Answer from the drawing. Dimensions are ordinates in mm from the lowest x, y and z of the part. Coordinates: 2 decimals unless noted, no trailing zeros. Write each loop counter-clockwise with the first axis right and the second up, starting at its lowest first coordinate (ties: lowest second). Pieces come first, ordered by that corner, then holes. Notation, with made-up numbers: (80, 1.25) - (91, 1.25) arc R32 ccw to (91, 30.25) - close; hole circle Ø1 at (83, -36.5). An arc over 180 degrees is marked (long way). Use one line per item in the form item = value. Start each with the question number.
Item 1: A cutting plane is placed at A-A (x = 38.1). Write down the section's boundary in (y, z).
Item 2: Given pin 1 (4 mm diameter, centred on x = 14, y = 26, fed in from -Z); pin 2 (3 mm diameter, centred on x = 67, z = 11, fed in from -Y); pin 3 (6 mm diameter, centred on x = 45, z = 32, fed in from +Y); pin 4 (12 mm diameter, centred on y = 47.5, z = 14, fed in from -X), each flat-ended and moving along its own axis, determine where each tip first touches the part or whether it passes through.
Item 3: A cutting plane is placed at B-B (z = 6). Write down the section's boundary in (x, y).
Item 4: Determine the mould class of the marked faces 1, 2 and 3 for opening direction X: released by +X, released by -X, zero draft, split by the parting line, or undercut.
Item 5: Consider probe 1 along Z at (x, y) = (23.5, 39); probe 2 along X at (y, z) = (38, 59); probe 3 along Y at (x, z) = (38.1, 60.25). Determine where each line is inside the solid, lowest interval first.
Item 6: A cutting plane is placed at C-C (z = 35). Write down the section's boundary in (x, y), then the cut area to 3 significant figures.
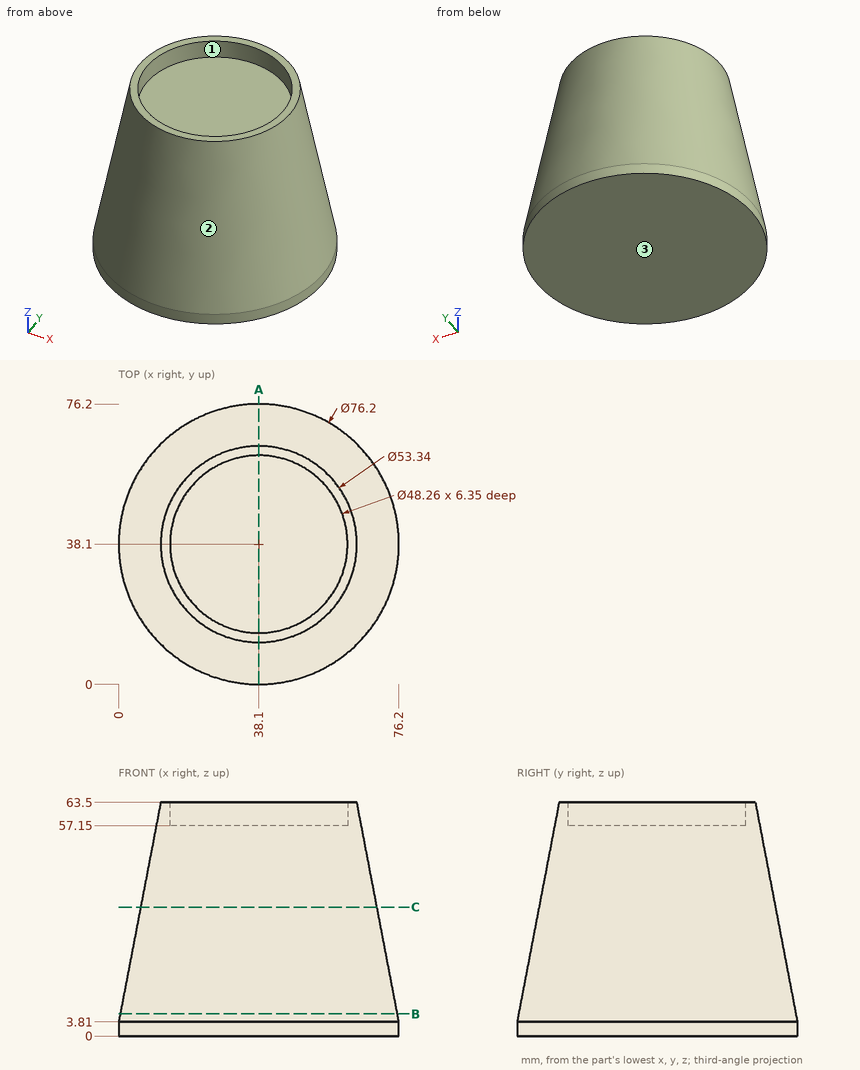
Answer:
q1.outline = (0, 0) - (76.2, 0) - (76.2, 3.81) - (64.77, 63.5) - (62.23, 63.5) - (62.23, 57.15) - (13.97, 57.15) - (13.97, 63.5) - (11.43, 63.5) - (0, 3.81) - close
q2.pin_1 = 0
q2.pin_2 = 13.59
q2.pin_3 = 70.87
q2.pin_4 = 1.49
q3.outline = circle Ø75.36 at (38.1, 38.1)
q4.face_1 = undercut
q4.face_2 = split by the parting line
q4.face_3 = zero draft
q5.probe_1 = 0 to 57.15
q5.probe_2 = 10.57 to 13.97, 62.23 to 65.63
q5.probe_3 = 10.81 to 13.97, 62.23 to 65.39
q6.outline = circle Ø64.25 at (38.1, 38.1)
q6.area = 3,240 mm²
